```python
from build123d import *

# Parameters (mm, degrees)
SKETCH_1_R               = 25
EXTRUDE_1_DEPTH          = 30
EXTRUDE_1_TAPER          = 10
SKETCH_3_W               = 20.3
SKETCH_3_H               = 20.3
CUT_EXTRUDE_2_DEPTH      = 47.36809265
CUT_EXTRUDE_3_DEPTH      = 53.540674891
CUT_EXTRUDE_3_DEPTH_BACK = 53.540674891
SKETCH_4_R               = 2.65
CUT_EXTRUDE_4_DEPTH      = 53.540674891
CUT_EXTRUDE_4_DEPTH_BACK = 53.540674891
SKETCH_5_R               = 2.65
CUT_EXTRUDE_START        = -15
SKETCH_6_R               = 4.5
CUT_EXTRUDE_5_DEPTH      = 19
SKETCH_7_R               = 4.5
CUT_EXTRUDE_6_DEPTH      = 19


with BuildPart() as part:
    # 草图1 → 凸台-拉伸1 (new body)
    with BuildSketch(Plane(origin=(0, 0, 0), x_dir=(1, 0, 0), z_dir=(0, 1, 0))):
        Circle(SKETCH_1_R)
    extrude(amount=EXTRUDE_1_DEPTH, taper=EXTRUDE_1_TAPER)

    # 草图3 → 切除-拉伸2 (cut, through all)
    with BuildSketch(Plane(origin=(0, 30, 0), x_dir=(1, 0, 0), z_dir=(0, 1, 0))):
        Rectangle(SKETCH_3_W, SKETCH_3_H)
    extrude(amount=-CUT_EXTRUDE_2_DEPTH, mode=Mode.SUBTRACT)

    # 草图4 → 切除-拉伸3 (cut, two sides: drawn at the far end of the back side and taken through both)
    with BuildSketch(Plane(origin=(-10.15, 0, 0), x_dir=(0, 0, -1), z_dir=(1, 0, 0)).offset(-CUT_EXTRUDE_3_DEPTH_BACK)):
        with Locations(Location((0, 20, 0), (0, 0, 301.069984195))):
            Circle(SKETCH_4_R)
    extrude(amount=CUT_EXTRUDE_3_DEPTH + CUT_EXTRUDE_3_DEPTH_BACK, mode=Mode.SUBTRACT)

    # 草图5 → 切除-拉伸4 (cut, two sides: drawn at the far end of the back side and taken through both)
    with BuildSketch(Plane(origin=(0, 0, 10.15), x_dir=(-1, 0, 0), z_dir=(0, 0, -1)).offset(-CUT_EXTRUDE_4_DEPTH_BACK)):
        with Locations((0, 20)):
            Circle(SKETCH_5_R)
    extrude(amount=CUT_EXTRUDE_4_DEPTH + CUT_EXTRUDE_4_DEPTH_BACK, mode=Mode.SUBTRACT)

    # 草图6 → 切除-拉伸5 (cut)
    with BuildSketch(Plane.XY.offset(-20.15).offset(CUT_EXTRUDE_START)):
        with Locations(Location((0, 20, 0), (0, 0, 224.651479051))):
            Circle(SKETCH_6_R)
    cut_extrude_5 = extrude(amount=CUT_EXTRUDE_5_DEPTH, mode=Mode.SUBTRACT)

    # 草图7 → 切除-拉伸6 (cut)
    with BuildSketch(Plane.ZY.offset(-20.15).offset(CUT_EXTRUDE_START)):
        with Locations(Location((0, 20, 0), (0, 0, 224.651479051))):
            Circle(SKETCH_7_R)
    cut_extrude_6 = extrude(amount=CUT_EXTRUDE_6_DEPTH, mode=Mode.SUBTRACT)

    # 镜向1: 切除-拉伸6 across plane
    add(cut_extrude_6.mirror(Plane.ZY.offset(-0.15)), mode=Mode.SUBTRACT)

    # 镜向2: 切除-拉伸5 across plane
    add(cut_extrude_5.mirror(Plane.XY.offset(-0.15)), mode=Mode.SUBTRACT)


solid = part.part
```
Work out the finished part from the listing and answer in its coordinate system (mm). A direction names the side the tool comes from. Give positions to 0.01 mm unless a question says otherwise; leave off trailing zeros. Loops run counter-clockwise (first coordinate to the right, second up) from the corner with the lowest first, then second, coordinate; pieces in that order, holes last. Notation, with made-up numbers: (38, 73.5) -> (79, 73.5) arc R13 ccw to (79, 97.5) -> close; hole circle Ø4 at (72, -22). An arc over 180 degrees is marked (long way). One line per question, with ' | ' between items. Start each with the question number.
1) Section C-C, the plane z = 0 is taken. State how many separate pieces and enclosed holes the cut face has, then the cut area to 3 significant figures.
2) Section A-A, the plane x = 0 is taken. Determine the outline of the cut face in (y, z), then the cut area to 3 significant figures.
3) For faces 5 (the face through (-10.15, 15, 0)), 6 (the face through (-18.39, 15.6, 0.95)), 7 (the face through (-3, 20, -16.15)), 8 (the face through (-3, 20, 15.85)), determine the directions among +Z, -Z, +X, -X, +Y, -Y from which every point of the face is accessible in a straight line to the end or side of a thin tool.
4) Section B-B, the plane y = 6 is taken. Determine the outline of the cut face in (x, z).
5) Straight lines are drawn through the part: L1, parallel to Y at x = -17.25, z = 0; L2, parallel to Y at x = 12.6, z = 0; L3, parallel to Z at x = 2, y = 17. For each, find the intervals that lie inside material, in ascending order.
6) Determine the mould class of faces 1 (the face through (0, 0, 11)), 2 (the face through (18.57, 15.6, 0.95)), 3 (the face through (0, 30, 13)), 4 (the face through (0, 15, 10.15)) for opening direction Y: +Y half, -Y half, draft (parallel to the pull), parting line (faces both ways), or undercut.
7) Each of these flat-tipped pins is pushed along its axis until it touches: pin 1 (1 mm diameter, centred on y = 11, z = 1, fed in from -X); pin 2 (11.5 mm diameter, centred on x = 0, y = 20, fed in from +Z); pin 3 (6 mm diameter, centred on y = 16.5, z = -11.5, fed in from +X). Where does it stop, or does it pass through?
Resolved:
1) separate pieces: 4 | enclosed holes: 0 | area: 572 mm2
2) outline: (0, -25) -> (15.5, -22.27) -> (15.5, -16.15) -> (17.35, -16.15) -> (17.35, -10.15) -> (0, -10.15) -> close; (0, 10.15) -> (17.35, 10.15) -> (17.35, 15.85) -> (15.5, 15.85) -> (15.5, 22.27) -> (0, 25) -> close; (22.65, -16.15) -> (24.5, -16.15) -> (24.5, -20.68) -> (30, -19.71) -> (30, -10.15) -> (22.65, -10.15) -> close; (22.65, 10.15) -> (30, 10.15) -> (30, 19.71) -> (24.5, 20.68) -> (24.5, 15.85) -> (22.65, 15.85) -> close | area: 572 mm2
3) face 5: +Y, -Y | face 6: -X | face 7: -Z | face 8: +Z
4) outline: circle Ø47.88 at (0, 0); hole (-10.15, -10.15) -> (10.15, -10.15) -> (10.15, 10.15) -> (-10.15, 10.15) -> close
5) L1: 0 to 15.5, 24.5 to 30 | L2: 0 to 17.35, 22.65 to 30 | L3: -16.15 to -10.15, 10.15 to 15.85
6) face 1: -Y half | face 2: undercut | face 3: +Y half | face 4: draft
7) pin 1: x = -23.13 | pin 2: z = 22.49 | pin 3: x = 20.51
